Autodesk Inventor part; units mm, degrees
ref_plane "YZ Plane" through (0, 0, 0) normal (1, 0, 0) x (0, 1, 0)
ref_plane "XZ Plane" through (0, 0, 0) normal (0, 1, 0) x (-1, 0, 0)
ref_plane "XY Plane" through (0, 0, 0) normal (0, 0, 1) x (1, 0, 0)
sketch "Sketch1" plane through (0, 0, 0) normal (0, 0, 1) x (1, 0, 0)
  line L0 (-114.3, 77.8543) -> (-127, 77.8543)
  line L1 (-127, 77.8543) -> (-163.2323, 36.0005)
  arc A0 (-163.2323, 36.0005) -> (-215.9, -105.3078) centre (0, -105.3078) ccw
  line L2 (-152.4, -105.3078) -> (-215.9, -105.3078)
  arc A1 (152.4, -105.3078) -> (-152.4, -105.3078) centre (0, -105.3078) ccw
  line L3 (215.9, -105.3078) -> (152.4, -105.3078)
  arc A2 (215.9, -105.3078) -> (163.2323, 36.0005) centre (0, -105.3078) ccw
  line L4 (163.2323, 36.0005) -> (127, 77.8543)
  line L5 (127, 77.8543) -> (114.3, 77.8543)
  line L6 (114.3, 77.8543) -> (114.3, 90.5543)
  line L7 (114.3, 90.5543) -> (46.5518, 105.5138)
  arc A3 (46.5518, 105.5138) -> (-46.5518, 105.5138) centre (0, -105.3078) ccw
  line L8 (-46.5518, 105.5138) -> (-114.3, 90.5543)
  line L9 (-114.3, 90.5543) -> (-114.3, 77.8543)
  circle A4 centre (-174.6359, -42.9949) radius 3.302
  circle A5 centre (-181.5133, -67.4461) radius 3.302
  circle A6 centre (-184.9846, -92.6078) radius 3.302
  circle A7 centre (-12.7, 63.1241) radius 3.302
  circle A8 centre (-37.8617, 76.2055) radius 3.302
  circle A9 centre (-62.0706, 51.784) radius 3.302
  circle A10 centre (12.7, 63.1241) radius 3.302
  circle A11 centre (62.0706, 51.784) radius 3.302
  circle A12 centre (62.3129, 69.3281) radius 3.302
  circle A13 centre (174.6359, -42.9949) radius 3.302
  circle A14 centre (164.6231, -67.4949) radius 3.302
  circle A15 centre (181.5133, -67.4461) radius 3.302
  circle A16 centre (184.9846, -92.6078) radius 3.302
  circle A17 centre (168.4319, -92.6078) radius 3.302
  circle A18 centre (157.0918, -43.2372) radius 3.302
  circle A19 centre (37.8617, 76.2055) radius 3.302
  circle A20 centre (37.8128, 59.3154) radius 3.302
  circle A21 centre (12.7, 79.6768) radius 3.302
  circle A22 centre (-62.3129, 69.3281) radius 3.302
  circle A23 centre (-37.8128, 59.3154) radius 3.302
  circle A24 centre (-12.7, 79.6768) radius 3.302
  circle A25 centre (-168.4319, -92.6078) radius 3.302
  circle A26 centre (-164.6231, -67.4949) radius 3.302
  circle A27 centre (-157.0918, -43.2372) radius 3.302
  line L10 (-127, 143.7166) -> (-127, -105.3078)
  line L11 (-127, -21.0655) -> (-127, 108.4537)
  line L12 (-142.24, -21.0655) -> (-142.24, 38.6612) construction
  circle A28 centre (-142.24, -7.2274) radius 3.302
  circle A29 centre (-142.24, 18.1726) radius 3.302
  line L13 (-157.48, -21.0655) -> (-157.48, 42.6453)
  line L14 (-127, -21.0655) -> (-157.48, -21.0655)
  line L15 (-127, 108.4537) -> (-131.3752, 105.9825)
  line L16 (-143.2518, 91.0321) -> (-157.48, 42.6453)
  arc A30 (-131.3752, 105.9825) -> (-143.2518, 91.0321) centre (-118.8834, 83.8665) ccw
  circle A31 centre (142.24, 14.8706) radius 3.302
  circle A32 centre (-142.24, 14.8706) radius 3.302
  circle A33 centre (-142.24, -10.5294) radius 3.302
  circle A34 centre (142.24, -10.5294) radius 3.302
  point P0 (0, 0)
  dimension "d1" = 6.604
  dimension "d2" = 6.604
  dimension "d3" = 25.4
  dimension "d6" = 15.24
  dimension "d7" = 15.24
  dimension "d8" = 25.4
extrude "Extrusion1" add sketch "Sketch1" along normal blind 3.175 contours L10 L14 L13 L1 | L1 L16 A30 L15 L10 | A28 A33 | A29 A32 picked at (-142.4059, -12.7065) picked at (-142.4059, 12.6935)
sketch "Sketch2" plane through (0, 0, 0) normal (0, 0, -1) x (-1, 0, 0)
  line L0 (127, -21.0655) -> (127, 108.4537)
  line L1 (157.48, 42.6453) -> (157.48, -21.0655)
  line L2 (127, -21.0655) -> (157.48, -21.0655)
  line L3 (157.48, -21.0655) -> (157.48, -15.2234)
  line L4 (157.48, -15.2234) -> (127, -15.2234)
  line L5 (127, -15.2234) -> (127, -21.0655)
  point P0 (0, 0)
extrude "Extrusion2" cut sketch "Sketch2" against normal blind 25.4
sketch "Sketch3" plane through (0, 0, 0) normal (0, 0, -1) x (-1, 0, 0)
  line L0 (127, -15.2234) -> (157.48, -15.2234)
  line L1 (157.48, 42.6453) -> (157.48, -15.2234)
  line L2 (143.2518, 91.0321) -> (157.48, 42.6453)
  arc A0 (143.2518, 91.0321) -> (131.3752, 105.9825) centre (118.8834, 83.8665) ccw
  line L3 (127, 108.4537) -> (131.3752, 105.9825)
  line L4 (127, -15.2234) -> (127, 108.4537)
  circle A1 centre (142.24, 18.1726) radius 3.302
  circle A2 centre (142.24, -7.2274) radius 3.302
  circle A3 centre (128.3509, -8.4471) radius 3.302
  line L5 (157.48, 42.6453) -> (157.48, -15.2234)
  line L6 (157.48, -15.2234) -> (127, -15.2234)
  line L7 (127, -15.2234) -> (127, -19.0291)
  line L8 (127, -19.0291) -> (157.48, -19.0291)
  line L9 (157.48, -19.0291) -> (157.48, -15.2234)
  circle A4 centre (25.4, 77.2006) radius 3.302
  circle A5 centre (50.4225, 72.8376) radius 3.302
  circle A6 centre (73.8239, 46.08) radius 3.302
  circle A7 centre (159.4716, -56.8709) radius 3.302
  circle A8 centre (155.1086, -31.8485) radius 3.302
  circle A9 centre (146.5122, -7.9473) radius 3.302
  circle A10 centre (137.9833, -107.1921) radius 3.302
  circle A11 centre (159.4716, -82.2709) radius 3.302
  circle A12 centre (146.5122, -131.1945) radius 3.302
  circle A13 centre (74.3236, -203.3832) radius 3.302
  circle A14 centre (25.4, -199.763) radius 3.302
  circle A15 centre (25.4, -216.3425) radius 3.302
  circle A16 centre (50.4225, -211.9795) radius 3.302
  circle A17 centre (50.3212, -194.8542) radius 3.302
  circle A18 centre (73.8239, -185.2218) radius 3.302
  circle A19 centre (155.1086, -107.2934) radius 3.302
  circle A20 centre (142.892, -82.2709) radius 3.302
  circle A21 centre (128.3509, -130.6948) radius 3.302
  circle A22 centre (128.3509, -8.4471) radius 3.302
  circle A23 centre (137.9833, -31.9498) radius 3.302
  circle A24 centre (142.892, -56.8709) radius 3.302
  circle A25 centre (74.3236, 64.2413) radius 3.302
  circle A26 centre (50.3212, 55.7124) radius 3.302
  circle A27 centre (25.4, 60.6211) radius 3.302
  arc A28 (12.7, -234.6709) -> (12.7, 95.5291) centre (12.7, -69.5709) ccw
  line L10 (12.7, 95.5291) -> (12.7, 44.7291)
  arc A29 (12.7, -183.8709) -> (12.7, 44.7291) centre (12.7, -69.5709) ccw
  line L11 (12.7, -183.8709) -> (12.7, -234.6709)
  line L12 (142.24, -19.0291) -> (127, 3.43)
  point P0 (0, 0)
extrude "Extrusion4" add sketch "Sketch3" against normal blind 3.175 contours L12 L4 A28 L1 L0 | L0 L9 L8 L12 | A28 L4 L3 A0 L2 L1 | A1 | A2 A9 | A9 A2 picked at (144.0113, -7.5677) picked at (141.8341, -7.293)
sketch "Sketch4" plane through (0, 0, 0) normal (0, 0, -1) x (-1, 0, 0)
  circle A0 centre (25.4, 77.2006) radius 3.302
  circle A1 centre (50.4225, 72.8376) radius 3.302
  circle A2 centre (73.8239, 46.08) radius 3.302
  circle A3 centre (159.4716, -56.8709) radius 3.302
  circle A4 centre (155.1086, -31.8485) radius 3.302
  circle A5 centre (146.5122, -7.9473) radius 3.302
  circle A6 centre (137.9833, -107.1921) radius 3.302
  circle A7 centre (159.4716, -82.2709) radius 3.302
  circle A8 centre (146.5122, -131.1945) radius 3.302
  circle A9 centre (74.3236, -203.3832) radius 3.302
  circle A10 centre (25.4, -199.763) radius 3.302
  circle A11 centre (25.4, -216.3425) radius 3.302
  circle A12 centre (50.4225, -211.9795) radius 3.302
  circle A13 centre (50.3212, -194.8542) radius 3.302
  circle A14 centre (73.8239, -185.2218) radius 3.302
  circle A15 centre (155.1086, -107.2934) radius 3.302
  circle A16 centre (142.892, -82.2709) radius 3.302
  circle A17 centre (128.3509, -130.6948) radius 3.302
  circle A18 centre (128.3509, -8.4471) radius 3.302
  circle A19 centre (137.9833, -31.9498) radius 3.302
  circle A20 centre (142.892, -56.8709) radius 3.302
  circle A21 centre (74.3236, 64.2413) radius 3.302
  circle A22 centre (50.3212, 55.7124) radius 3.302
  circle A23 centre (25.4, 60.6211) radius 3.302
  arc A24 (12.7, -234.6709) -> (12.7, 95.5291) centre (12.7, -69.5709) ccw
  line L0 (12.7, 95.5291) -> (12.7, 44.7291)
  arc A25 (12.7, -183.8709) -> (12.7, 44.7291) centre (12.7, -69.5709) ccw
  line L1 (12.7, -183.8709) -> (12.7, -234.6709)
  line L2 (127, -15.2234) -> (127, 108.4537)
  line L3 (127, -15.2234) -> (139.6576, -15.2234)
  line L4 (139.6576, -15.2234) -> (142.24, -19.0291)
  line L5 (142.24, -19.0291) -> (157.48, -19.0291)
  line L6 (157.48, 42.6453) -> (157.48, -19.0291)
  line L7 (143.2518, 91.0321) -> (157.48, 42.6453)
  arc A26 (143.2518, 91.0321) -> (131.3752, 105.9825) centre (118.8834, 83.8665) ccw
  line L8 (127, 108.4537) -> (131.3752, 105.9825)
  line L9 (127, -15.2234) -> (139.6576, -15.2234)
  line L10 (142.24, -19.0291) -> (139.6576, -15.2234)
  line L11 (142.24, -19.0291) -> (127, 8.7406)
  line L12 (127, -15.2234) -> (127, 108.4537)
  line L13 (142.24, -19.0291) -> (123.8625, -20.0167)
  line L14 (123.8625, -20.0167) -> (123.8625, 8.7406)
  line L15 (123.8625, 8.7406) -> (127, 8.7406)
  circle A27 centre (12.7, -69.5709) radius 147.32
  circle A28 centre (134.1655, 26.6191) radius 3.302
  point P0 (0, 0)
  dimension "d17" = 6.604
  dimension "d18" = 154.94
extrude "Extrusion5" cut sketch "Sketch4" against normal blind 6.604 contours L11 L4 L3 L2 A18 | A18 L2 | A28 picked at (128.551, -8.4471)
sketch "Sketch5" plane through (0, 0, 0) normal (0, 0, -1) x (-1, 0, 0)
  circle A0 centre (25.4, 77.2006) radius 3.302
  circle A1 centre (50.4225, 72.8376) radius 3.302
  circle A2 centre (73.8239, 46.08) radius 3.302
  circle A3 centre (159.4716, -56.8709) radius 3.302
  circle A4 centre (155.1086, -31.8485) radius 3.302
  circle A5 centre (146.5122, -7.9473) radius 3.302
  circle A6 centre (137.9833, -107.1921) radius 3.302
  circle A7 centre (159.4716, -82.2709) radius 3.302
  circle A8 centre (146.5122, -131.1945) radius 3.302
  circle A9 centre (74.3236, -203.3832) radius 3.302
  circle A10 centre (25.4, -199.763) radius 3.302
  circle A11 centre (25.4, -216.3425) radius 3.302
  circle A12 centre (50.4225, -211.9795) radius 3.302
  circle A13 centre (50.3212, -194.8542) radius 3.302
  circle A14 centre (73.8239, -185.2218) radius 3.302
  circle A15 centre (155.1086, -107.2934) radius 3.302
  circle A16 centre (142.892, -82.2709) radius 3.302
  circle A17 centre (128.3509, -130.6948) radius 3.302
  circle A18 centre (128.3509, -8.4471) radius 3.302
  circle A19 centre (137.9833, -31.9498) radius 3.302
  circle A20 centre (142.892, -56.8709) radius 3.302
  circle A21 centre (74.3236, 64.2413) radius 3.302
  circle A22 centre (50.3212, 55.7124) radius 3.302
  circle A23 centre (25.4, 60.6211) radius 3.302
  arc A24 (12.7, -234.6709) -> (12.7, 95.5291) centre (12.7, -69.5709) ccw
  line L0 (12.7, 95.5291) -> (12.7, 44.7291)
  arc A25 (12.7, -183.8709) -> (12.7, 44.7291) centre (12.7, -69.5709) ccw
  line L1 (12.7, -183.8709) -> (12.7, -234.6709)
  point P0 (0, 0)
extrude "Extrusion6" cut sketch "Sketch5" against normal blind 6.604 contours A5
fillet "Fillet1" radius 6.35 1 edges at (-127, 8.7406, 1.5875)
sketch "Sketch6" plane through (0, 0, 3.175) normal (0, 0, 1) x (1, 0, 0)
  circle A0 centre (-128.3509, -8.4471) radius 3.302
  arc A1 (-127.7832, 7.3135) -> (-127, 10.3686) centre (-133.35, 10.3686) ccw
  line L0 (-127, 10.3686) -> (-127, 108.4537)
  line L1 (-127, 108.4537) -> (-131.3752, 105.9825)
  arc A2 (-131.3752, 105.9825) -> (-143.2518, 91.0321) centre (-118.8834, 83.8665) ccw
  line L2 (-143.2518, 91.0321) -> (-157.48, 42.6453)
  line L3 (-157.48, 42.6453) -> (-157.48, -19.0291)
  line L4 (-157.48, -19.0291) -> (-142.24, -19.0291)
  line L5 (-142.24, -19.0291) -> (-127.7832, 7.3135)
  circle A3 centre (-146.5122, -7.9473) radius 3.302
  circle A4 centre (-134.1655, 26.6191) radius 3.302
  line L6 (-127.7832, 7.3135) -> (-142.24, -19.0291)
  line L7 (-142.24, -19.0291) -> (-120.3644, -19.0291)
  line L8 (-127, 10.3686) -> (-127, 108.4537)
  line L9 (-127, 10.3686) -> (-120.3644, -9.1547)
  line L10 (-120.3644, -9.1547) -> (-120.3644, -19.0291)
  line L11 (-142.24, -19.0291) -> (-127, 10.3686)
  point P0 (0, 0)
extrude "Extrusion7" add sketch "Sketch6" against normal blind 3.175 contours A1 L9 L10 L7 L5
equation "\"d19\" = d17"
equation "\"d21\" = d17"
properties part number "13in coil holder plate" material "PVC-Piping"
The model under review builds one solid part; all positions refer to its coordinate system, in mm. A direction names the side the tool comes from. Round coordinates to 2 decimals unless told otherwise and drop trailing zeros. Order: outer loops, then holes, each group sorted by start corner. A loop starts at its lowest first (then second) coordinate and runs counter-clockwise, first axis right, second up. Notation, with made-up numbers: M 65,-19 L 102,-19 A17 ccw 102,11 Z; hole C 69,59 d6. An arc over 180 degrees is marked long. Use a Markdown table: item, result.
1) Wall thickness on line 1 along X through (y, z) = (26.5, 1.15); line 2 along X through (y, z) = (-5.5, 0.6); line 3 along X through (y, z) = (-8.5, 2.4): over which ranges is each line inside the solid? List them lowest first. Write a range as [from, to].
Report:
| item | result |
|---|---|
| line 1 | [-157.48, -137.47], [-130.87, -127] |
| line 2 | [-157.48, -148.73], [-144.3, -129.84], [-126.86, -121.61] |
| line 3 | [-157.48, -149.77], [-143.26, -131.65], [-125.05, -120.59] |
2) Consider section A-A (x = -145.5). Write out the cut boundary in (y, z) (1 decimal).
Report:
| item | result |
|---|---|
| outline | M -19,0 L -11.1,0 L -11.1,3.2 L -19,3.2 Z; M -4.8,0 L 83.4,0 L 83.4,3.2 L -4.8,3.2 Z |
3) Consider section D-D (x = -134). Write out the cut boundary in (y, z) (3 decimals).
Report:
| item | result |
|---|---|
| outline | M -19.029,0 L 23.321,0 L 23.321,3.175 L -19.029,3.175 Z; M 29.917,0 L 104.279,0 L 104.279,3.175 L 29.917,3.175 Z |
4) Consider section B-B (z = 2.6). Write out the cut boundary in (x, y).
Report:
| item | result |
|---|---|
| outline | M -157.48,-19.03 L -120.36,-19.03 L -120.36,-9.15 L -127,10.37 L -127,108.45 L -131.38,105.98 A25.4 ccw -143.25,91.03 L -157.48,42.65 Z; hole C -146.51,-7.95 d6.6; hole C -134.17,26.62 d6.6; hole C -128.35,-8.45 d6.6 |
5) Draft analysis for pull direction Y (two halves, no side actions). For faces 3 (the face through (-123.729, 0.744, 1.61)), 4 (the face through (-139, -19.029, 2)), 5 (the face through (-130.867, 26.764, 1.565)), state which applies: released by +Y, released by -Y, zero draft, split by the parting line, or undercut.
Report:
| item | result |
|---|---|
| face 3 | released by +Y |
| face 4 | released by -Y |
| face 5 | undercut |
6) Consider section C-C (y = 36). Write out the cut boundary in (x, z) (3 decimals).
Report:
| item | result |
|---|---|
| outline | M -157.48,0 L -127,0 L -127,3.175 L -157.48,3.175 Z |
7) Insertion check: pin 1 (1.6 mm diameter, centred on y = 55.5, z = 1, fed in from +X). The pin has a flat end and moves straight along its axis. Give the tip position at first contact, or say it passes through.
Report:
| item | result |
|---|---|
| pin 1 | x = -127 |
8) Tool access review of faces 1 (the face through (-127, 60, 2)), 2 (the face through (-120.364, -14, 2)): name each direction out of +Z, -Z, +X, -X, +Y, -Y from which nothing blocks a thin tool from reaching the whole face with its end or side.
Report:
| item | result |
|---|---|
| face 1 | +Z, -Z, +X, +Y |
| face 2 | +Z, -Z, +X, +Y, -Y |
